Source: CAD feature listing. Evaluate the final solid. Frame: model axes, mm. Face numbers are marked on the shaded views. Give positions to 0.01 mm unless a question says otherwise; leave off trailing zeros. Loops run counter-clockwise (first coordinate to the right, second up) from the corner with the lowest first, then second, coordinate; pieces in that order, holes last. Notation, with made-up numbers: M 14,-16 L 38,-16 A24 cw 38,5 Z; hole C 39,48.25 d5. An arc over 180 degrees is marked long. Write item = value, one per line.
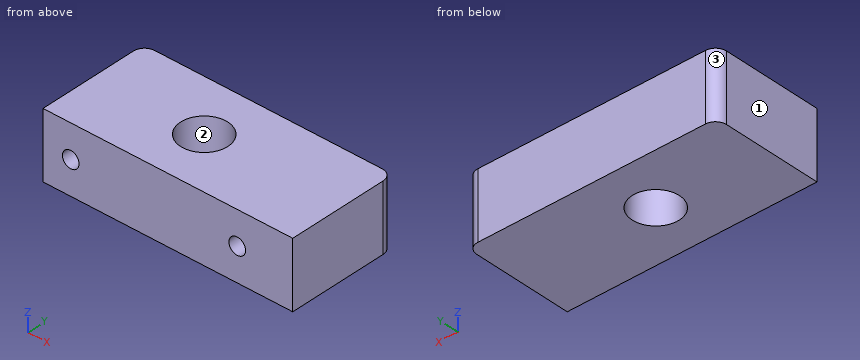
from build123d import *

# Parameters (mm, degrees)
SKETCH1_W           = 45
SKETCH1_H           = 20
SKETCH1_R           = 4.25
BOSS_EXTRUDE1_DEPTH = 12
FILLET1_R           = 2
SKETCH2_R           = 1.5
CUT_EXTRUDE1_DEPTH  = 5


with BuildPart() as part:
    # Sketch1 → Boss-Extrude1 (new body)
    with BuildSketch(Plane.XY):
        with Locations((22.5, 10)):
            Rectangle(SKETCH1_W, SKETCH1_H)
        with Locations((20, 10)):
            Circle(SKETCH1_R, mode=Mode.SUBTRACT)
    extrude(amount=BOSS_EXTRUDE1_DEPTH)

    # Fillet1
    fillet1_edges = [part.edges().sort_by_distance(p)[0] for p in [
        (0, 20, 6),
        (45, 20, 6),
    ]]
    fillet(fillet1_edges, radius=FILLET1_R)

    # Sketch2 → Cut-Extrude1 (cut)
    with BuildSketch(Plane.XZ):
        with Locations(Location((5, 6, 0), (0, 0, 270))):
            Circle(SKETCH2_R)
        with Locations(Location((35, 6, 0), (0, 0, 270))):
            Circle(SKETCH2_R)
    extrude(amount=-CUT_EXTRUDE1_DEPTH, mode=Mode.SUBTRACT)


solid = part.part
1. First-contact query: pin 1 Ø6 at (x, y) = (8.5, 13.5) entering from -Z; pin 2 Ø7 at (x, y) = (20, 10) entering from +Z. Flat tips, straight axial feed; report the tip coordinate or a pass-through.
Derived:
pin_1 = 0
pin_2 = through
2. Cut plane B-B, the plane y = 10. Return the cut outline in (x, z).
Derived:
outline = M 0,0 L 15.75,0 L 15.75,12 L 0,12 Z; M 24.25,0 L 45,0 L 45,12 L 24.25,12 Z
3. Material intervals for probe 1 along Y at (x, z) = (20, 7.25); probe 2 along X at (y, z) = (2.6, 6); probe 3 along Y at (x, z) = (16.5, 10.25), sorted ascending. Write a range as from..to.
Derived:
probe_1 = 0..5.75, 14.25..20
probe_2 = 0..3.5, 6.5..33.5, 36.5..45
probe_3 = 0..7.59, 12.41..20
4. Pull-direction query (Y, two-part tool) for the marked faces 1, 2 and 3; classes: +Y half, -Y half, draft (parallel to the pull), parting line (faces both ways), or undercut.
Derived:
face_1 = draft
face_2 = undercut
face_3 = +Y half
5. Cut plane A-A, the plane z = 2.5. Return the cut outline in (x, y), then the cut area to 3 significant figures.
Derived:
outline = M 0,0 L 45,0 L 45,18 A2 ccw 43,20 L 2,20 A2 ccw 0,18 Z; hole C 20,10 d8.5
area = 842 mm²
6. Cut plane C-C, the plane x = 5. Return the cut outline in (y, z), then the cut area to 3 significant figures.
Derived:
outline = M 0,0 L 20,0 L 20,12 L 0,12 L 0,7.5 L 5,7.5 L 5,4.5 L 0,4.5 Z
area = 225 mm²
7. Cut plane D-D, the plane x = 17.5. Return the cut outline in (y, z).
Derived:
outline = M 0,0 L 6.56,0 L 6.56,12 L 0,12 Z; M 13.44,0 L 20,0 L 20,12 L 13.44,12 Z
